from build123d import *

# Parameters (mm, degrees)
F3_R     = 25
F3_R_2   = 1.2
F4_DEPTH = 3


with BuildPart() as f1:
    # F0 (on Right) → F1 (revolve)
    with BuildSketch(Plane.YZ):
        Polygon((2, 25), (-3, 25), (-3, 24), (1, 21), (2, 21), align=None)
    revolve(axis=Axis((0, 1.602868, 0), (0, -1, 0)))

    # F3 (on offset) → F4 (join)
    with BuildSketch(Plane.XZ.offset(1)):
        with BuildLine():
            ThreePointArc((26.731818, 6.454448), (17.011065, 21.607259), (0, 27.5))
            Line((0, 27.5), (-27.5, 27.5))
            Line((-27.5, 27.5), (-27.5, 0))
            ThreePointArc((-27.5, 0), (-21.607259, -17.011065), (-6.454448, -26.731818))
            ThreePointArc((-6.454448, -26.731818), (-3.786128, -27.238121), (-1.080879, -27.47875))
            ThreePointArc((-1.080879, -27.47875), (0, -26.8), (1.080879, -27.47875))
            ThreePointArc((1.080879, -27.47875), (3.786128, -27.238121), (6.454448, -26.731818))
            ThreePointArc((6.454448, -26.731818), (19.445436, -19.445436), (26.731818, -6.454448))
            ThreePointArc((26.731818, -6.454448), (27.238121, -3.786128), (27.47875, -1.080879))
            ThreePointArc((27.47875, -1.080879), (26.8, 0), (27.47875, 1.080879))
            ThreePointArc((27.47875, 1.080879), (27.238121, 3.786128), (26.731818, 6.454448))
        make_face()
        Circle(F3_R, mode=Mode.SUBTRACT)
        with Locations((-20, 20)):
            Circle(F3_R_2, mode=Mode.SUBTRACT)
        with BuildLine():
            ThreePointArc((26.731818, -6.454448), (34, 0), (26.731818, 6.454448))
            ThreePointArc((26.731818, 6.454448), (27.238121, 3.786128), (27.47875, 1.080879))
            ThreePointArc((27.47875, 1.080879), (28.638161, 1.016243), (29.2, 0))
            ThreePointArc((29.2, 0), (28.638161, -1.016243), (27.47875, -1.080879))
            ThreePointArc((27.47875, -1.080879), (27.238121, -3.786128), (26.731818, -6.454448))
        make_face()
        with BuildLine():
            ThreePointArc((-1.080879, -27.47875), (-3.786128, -27.238121), (-6.454448, -26.731818))
            ThreePointArc((-6.454448, -26.731818), (0, -34), (6.454448, -26.731818))
            ThreePointArc((6.454448, -26.731818), (3.786128, -27.238121), (1.080879, -27.47875))
            ThreePointArc((1.080879, -27.47875), (1.169841, -27.732656), (1.2, -28))
            ThreePointArc((1.2, -28), (-0.267344, -29.169841), (-1.080879, -27.47875))
        make_face()
    extrude(amount=-F4_DEPTH)


solid = f1.part
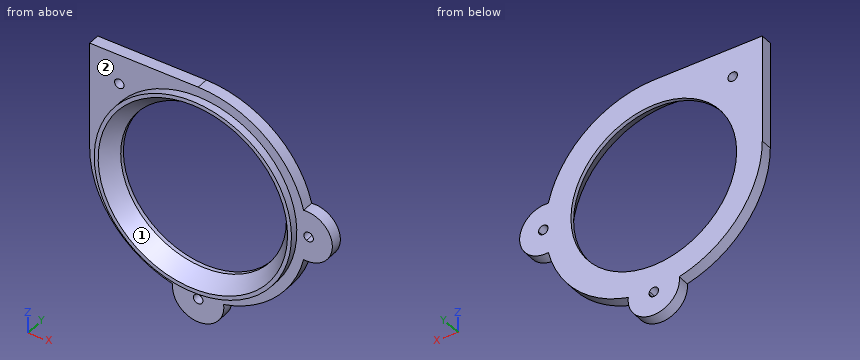
CAD build for the part. Positions are in the model's coordinates, mm. Face numbers are marked on the shaded views. Give positions to 0.01 mm unless a question says otherwise; leave off trailing zeros. Answer in a Markdown table with one row per item.
1. Probe probe 1 along Z at (x, y) = (-0.5, 1.7); probe 2 along X at (y, z) = (1.1, 4); probe 3 along Z at (x, y) = (3, 1.15). List the from-to ranges inside material, lowest first. Write a range as [from, to].
Data:
| item | result |
|---|---|
| probe 1 | z = [-33.98, -29.09], [-26.91, -20.99], [20.99, 27.5] |
| probe 2 | x = [-27.5, -20.62], [20.62, 32.62] |
| probe 3 | z = [-33.27, -20.78], [20.78, 27.34] |
2. Pull direction Z, two halves, no side cores. Call the marked faces 1 and 2: pulls with the +Z half, pulls with the -Z half, needs draft (parallel to the pull), parting line crosses it, or undercut.
Data:
| item | result |
|---|---|
| face 1 | undercut |
| face 2 | needs draft |
3. Saw through at A-A, the plane x = -20. Count the separate pieces of the cut face and the enclosed holes in it, plus the area to 3 significant figures.
Data:
| item | result |
|---|---|
| separate pieces | 3 |
| enclosed holes | 0 |
| area | 97.8 mm² |
4. Flat gauge pins, fed straight in: pin 1 (1.5 mm diameter, centred on y = -0.5, z = 14, fed in from +X); pin 2 (1.5 mm diameter, centred on y = -1, z = 11, fed in from +X); pin 3 (3 mm diameter, centred on y = -1, z = -7.5, fed in from -X). Where does each tip first touch, or does it go through?
Data:
| item | result |
|---|---|
| pin 1 | stops at x = 24.1 |
| pin 2 | stops at x = 25.52 |
| pin 3 | stops at x = -26.84 |
